Check sheet for the drawn part. Datum: minimum x, y, z corner. Units: mm. Give positions to 0.01 mm unless a question says otherwise; leave off trailing zeros. Loops run counter-clockwise (first coordinate to the right, second up) from the corner with the lowest first, then second, coordinate; pieces in that order, holes last.
1. Release check for a two-part mould opening along Z. For the marked faces 1, 2 and 3 record: +Z half, -Z half, draft (parallel to the pull), parting line (faces both ways), or undercut.
2. Cross-section at B-B, the plane y = 2.75. Record the cut outline in (x, z), plus the area to 3 significant figures.
3. Cross-section at A-A, the plane x = 19.9. Record the cut outline in (y, z), plus the area to 3 significant figures.
4. Cross-section at C-C, the plane x = 14.75. Record the cut outline in (y, z).
5. Cross-section at D-D, the plane z = 13.5. Record the cut outline in (x, y), plus the area to 3 significant figures.
6. Material ranges on L1, parallel to X at y = 2.55, z = 3.1; L2, parallel to Z at x = 19.9, y = 2.9; L3, parallel to Y at x = 5.75, z = 19, recorded low to high.
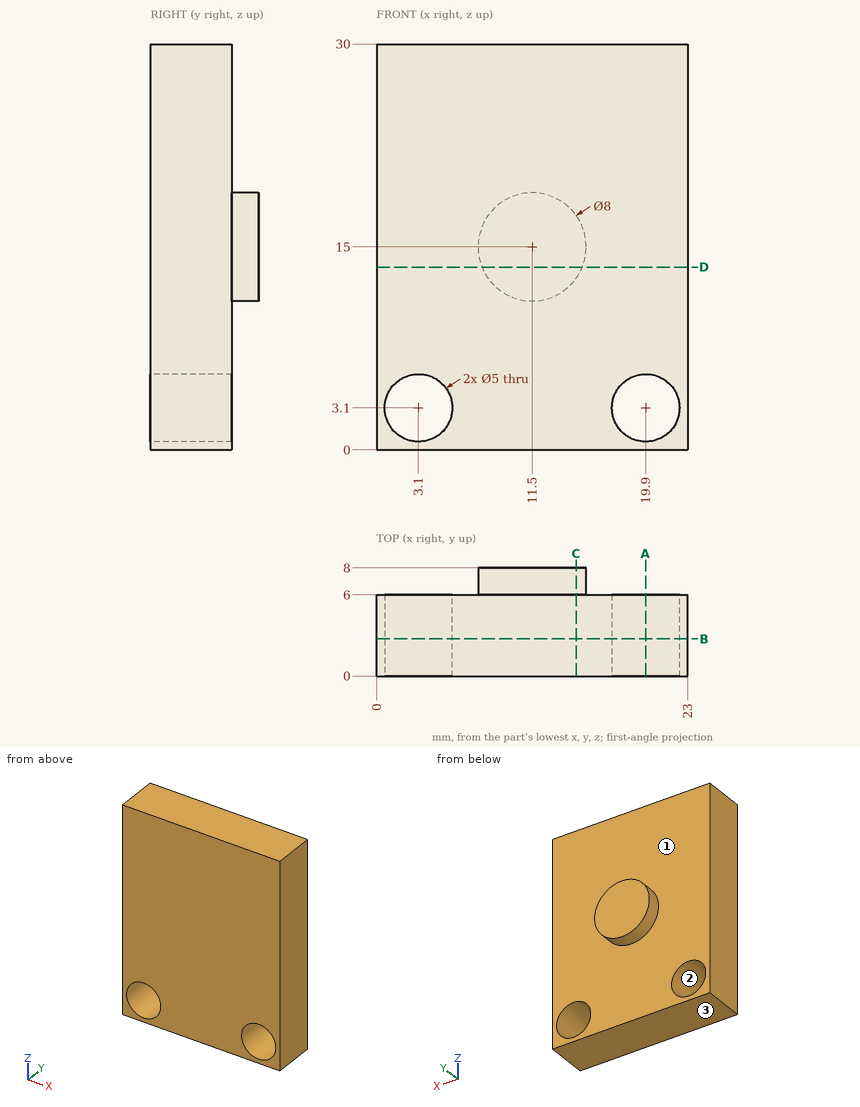
Result:
1. face 1: draft
1. face 2: undercut
1. face 3: -Z half
2. outline: (0, 0) - (23, 0) - (23, 30) - (0, 30) - close; hole circle Ø5 at (3.1, 3.1); hole circle Ø5 at (19.9, 3.1)
2. area: 651 mm2
3. outline: (0, 0) - (6, 0) - (6, 0.6) - (0, 0.6) - close; (0, 5.6) - (6, 5.6) - (6, 30) - (0, 30) - close
3. area: 150 mm2
4. outline: (0, 0) - (6, 0) - (6, 12.67) - (8, 12.67) - (8, 17.33) - (6, 17.33) - (6, 30) - (0, 30) - close
5. outline: (0, 0) - (23, 0) - (23, 6) - (15.21, 6) - (15.21, 8) - (7.79, 8) - (7.79, 6) - (0, 6) - close
5. area: 153 mm2
6. L1: x = 0 to 0.6, 5.6 to 17.4, 22.4 to 23
6. L2: z = 0 to 0.6, 5.6 to 30
6. L3: y = 0 to 6
